Here's the drawing with two shaded views (mm, measured from the low corner). I have some questions. A direction names the side the tool comes from. Give positions to 0.01 mm unless a question says otherwise; leave off trailing zeros. Loops run counter-clockwise (first coordinate to the right, second up) from the corner with the lowest first, then second, coordinate; pieces in that order, holes last. Notation, with made-up numbers: (8, 8) - (39, 8) arc R35 cw to (39, 44) - close; hole circle Ø3 at (-31, 49). An arc over 180 degrees is marked (long way). Use one line per item in the form item = value.
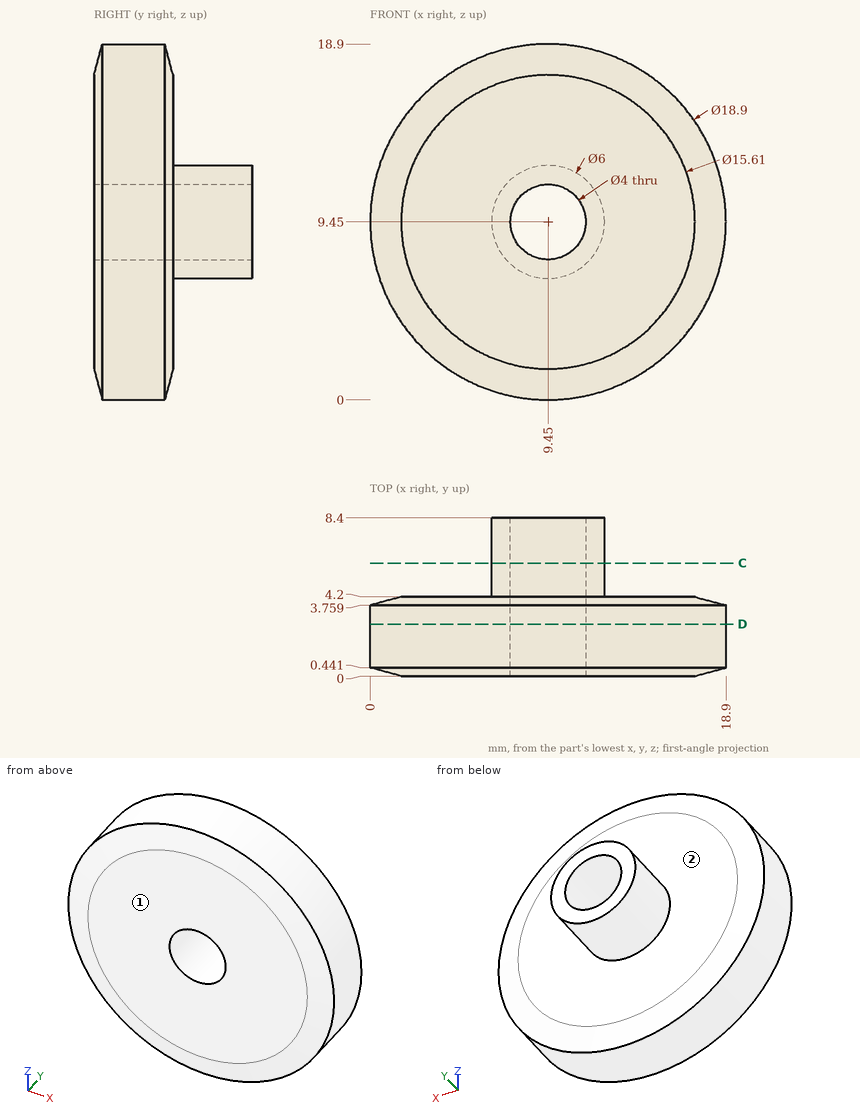
(1) For the marked faces 1 and 2, which set-ups out of +Z, -Z, +X, -X, +Y, -Y let a thin tool reach every point of the face, with its end or its side?
Geometry says:
face_1 = +Z, -Z, +X, -X, -Y
face_2 = +Y
(2) If we section it at D-D (y = 2.75): List the corners of the cut face in (x, z) for me.
Geometry says:
outline = circle Ø18.9 at (9.45, 9.45); hole circle Ø4 at (9.45, 9.45)
(3) If I drill on probe 1 along Z at (x, y) = (9.45, 5.75); probe 2 along Z at (x, y) = (9.45, 3.25); probe 3 along Y at (x, z) = (12, 11.5), over which ranges is the centre line in solid material (lowest first)?
Geometry says:
probe_1 = 6.45 to 7.45, 11.45 to 12.45
probe_2 = 0 to 7.45, 11.45 to 18.9
probe_3 = 0 to 4.2
(4) For P1, Ø2, axis at y = 6.5, z = 11, coming from the -X side; P2, Ø3, axis at y = 3, z = 8.5, coming from the -X side; P3, Ø2, axis at x = 8.5, z = 17, coming from the +Y side, each with a flat end and sliding along its axis, tell me the tip position at first contact or that it passes through.
Geometry says:
P1 = 6.5
P2 = 0
P3 = 4.2
(5) If we section it at C-C (y = 6): List the corners of the cut face in (x, z) for me.
Geometry says:
outline = circle Ø6 at (9.45, 9.45); hole circle Ø4 at (9.45, 9.45)
